Autodesk Inventor part; units mm, degrees
ref_plane "Płaszczyzna konstrukcyjna2" through (0, -40.4465, 0) normal (0, -1, 0) x (1, 0, 0)
ref_plane "YZ Plane" through (0, 0, 0) normal (1, 0, 0) x (0, 1, 0)
ref_plane "XZ Plane" through (0, 0, 0) normal (0, 1, 0) x (-1, 0, 0)
sketch "Szkic6" plane through (0, 0, 0) normal (0, 0, 1) x (1, 0, 0)
  line L0 (-29.6067, 0) -> (35.2678, 0) construction
  line L1 (0, 42.3419) -> (0, -58.3726) construction
  arc A0 (16.7535, 0) -> (0, -40.4465) centre (57.2, -40.4465) ccw
  line L2 (0, -40.4465) -> (57.2, -40.4465) construction
  line L3 (57.2, -40.4465) -> (10.8611, 5.8924) construction
  line L4 (16.7535, 0) -> (30.0596, 13.3061)
  line L5 (0, -40.4465) -> (0, -59.2641)
  point P0 (0, 0)
  dimension "d24" = 57.2
  dimension "d31" = 45
  dimension "d36" = 18.8176
  dimension "d37" = 18.8176
ref_plane "Płaszczyzna konstrukcyjna2" through (0, -40.4465, 0) normal (0, -1, 0) x (1, 0, 0)
sketch "Szkic8" plane through (0, -40.4465, 0) normal (0, -1, 0) x (1, 0, 0)
  circle A0 centre (0, 0) radius 19.05
  circle A1 centre (0, 0) radius 17.45
  dimension "d32" = 38.1
  dimension "d33" = 1.6
sweep "Przeciągnięcie2" add profiles "Szkic8" path "Szkic6"
equation "\"d32\" = OD"
equation "\"d33\" = THK"
equation "\"d24\" = R"
equation "\"d31\" = KAT"
equation "\"d36\" = PROSTKA"
equation "\"d37\" = PROSTKA"
equation "\"SzerokośćGięciaPodcięcia\" = Grubość"
equation "\"RozmiarPodcięciaNarożnika\" = 4 * Grubość"
equation "\"PromieńPrzejścia\" = PromieńGięcia"
equation "\"Rozmiar_promienia_Jacobiego\" = PromieńGięcia"
equation "\"Wielk_odstępu\" = Grubość"
equation "\"d2\" = PromieńGięcia"
equation "\"d23\" = PromieńGięcia"
equation "\"R\" = 57.2"
equation "\"OD\" = 38.1"
equation "\"THK\" = 1.6"
equation "\"KAT\" = 45deg"
equation "\"PROSTKA\" = 18.81761"
properties part number "Kolano 45° ø38,1x1,6 R57,2" material "304L"
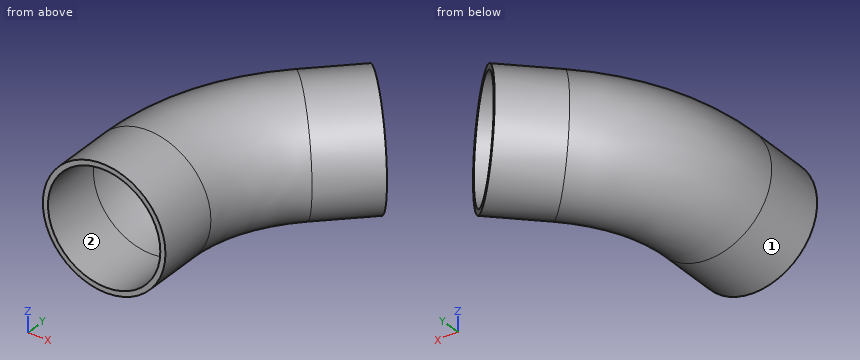
Source: CAD feature listing. Evaluate the final solid. Frame: model axes, mm. Face numbers are marked on the shaded views. Coordinates: 2 decimals unless noted, no trailing zeros. Write each question's results on one line, items separated by ' | '. Start each with the question number.
Item 1: Line query: probe 1 along Z at (x, y) = (0, -54); probe 2 along Z at (x, y) = (7.5, -25.5); probe 3 along X at (y, z) = (-0.5, 0). Output: solid intervals per line, ascending.
Item 2: Draft query along Z for the marked faces 1 and 2. Return one class per face: pulls with the +Z half, pulls with the -Z half, needs draft (parallel to the pull), parting line crosses it, or undercut.
Item 3: First-contact query: pin 1 Ø2 at (y, z) = (-44.5, 10) entering from -X; pin 2 Ø2 at (x, z) = (36.5, 5) entering from +Y; pin 3 Ø1 at (y, z) = (-49.5, -7) entering from +X. Flat tips, straight axial feed; report the tip coordinate or a pass-through.
Checked values:
1) probe 1: z = -19.05 to -17.45, 17.45 to 19.05 | probe 2: z = -18.3 to -16.63, 16.63 to 18.3 | probe 3: x = -7.75 to -5.86, 40.93 to 43.19
2) face 1: parting line crosses it | face 2: undercut
3) pin 1: stops at x = -16.79 | pin 2: stops at y = -2.8 | pin 3: stops at x = 17.91
